Can you work these out from the model? Positions are in its coordinate system, mm. Face numbers are marked on the shaded views. A direction names the side the tool comes from. Coordinates: 2 decimals unless noted, no trailing zeros. Write each loop counter-clockwise with the first axis right and the second up, starting at its lowest first coordinate (ties: lowest second). Pieces come first, ordered by that corner, then holes. Notation, with made-up numbers: (33, 71.5) - (68, 71.5) arc R24 ccw to (68, 103.5) - close; hole circle Ø11 at (55, 56.5). An arc over 180 degrees is marked (long way). One line per question, with ' | ' between items. Start each with the question number.
from build123d import *

# Parameters (mm, degrees)
SKETCH1_W                  = 231.4
SKETCH1_H                  = 30
BOSS_EXTRUDE1_DEPTH        = 3
BOSS_EXTRUDE2_DEPTH        = 3
F_8_0_8_DIAMETER_HOLE1_D   = 8
F_10_0_10_DIAMETER_HOLE1_D = 10
F_6_0_6_DIAMETER_HOLE1_D   = 6


with BuildPart() as part:
    # Sketch1 → Boss-Extrude1 (new body)
    with BuildSketch(Plane.XY):
        with Locations((0, -15)):
            Rectangle(SKETCH1_W, SKETCH1_H)
    extrude(amount=BOSS_EXTRUDE1_DEPTH)

    # Sketch2 → Boss-Extrude2 (add)
    with BuildSketch(Plane(origin=(0, 0, 0), x_dir=(1, 0, 0), z_dir=(0, 1, 0))):
        Polygon((-115.7, -3), (115.7, -3), (85.7, -33), (-85.7, -33), align=None)
    extrude(amount=-BOSS_EXTRUDE2_DEPTH)

    # Ø8.0 (8) Diameter Hole1 (through all)
    with Locations(Plane(origin=(0, 0, 0), x_dir=(-1, 0, 0), z_dir=(0, 0, -1))):
        with Locations((-100.7, -15), (100.7, -15)):
            Hole(F_8_0_8_DIAMETER_HOLE1_D / 2)

    # Ø10.0 (10) Diameter Hole1 (through all)
    with Locations(Plane(origin=(0, 0, 0), x_dir=(-1, 0, 0), z_dir=(0, 0, -1))):
        with Locations((62.5, -15)):
            Hole(F_10_0_10_DIAMETER_HOLE1_D / 2)

    # Ø6.0 (6) Diameter Hole1 (through all)
    with Locations(Plane(origin=(0, 0, 0), x_dir=(1, 0, 0), z_dir=(0, 1, 0))):
        with Locations((0, -18)):
            Hole(F_6_0_6_DIAMETER_HOLE1_D / 2)


solid = part.part
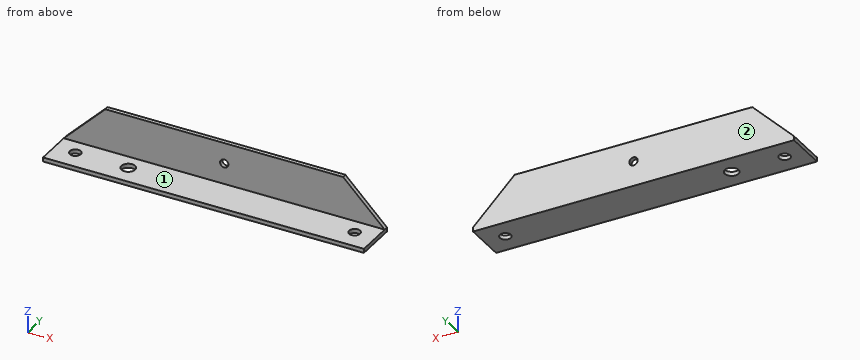
(1) I'm going to push flat-ended pins straight in: pin 1 (16 mm diameter, centred on x = -62.5, y = -15, fed in from +Z); pin 2 (12 mm diameter, centred on x = -55, z = 13.5, fed in from -Y). Where does each tip first touch, or does it pass through?
(2) If we section it at B-B on x = 0: List the corners of the cut face in (y, z) for me, plus the area to 3 significant figures.
(3) Which directions (+Z, -Z, +X, -X, +Y, -Y) give clear straight access to the entire face, cutting with the end or side of a thin tool? Please do the marked faces 1 and 2.
(4) If we section it at A-A on z = 18: List the corners of the cut face in (x, y) for me, plus the area to 3 significant figures.
(5) If I drill on probe 1 along Z at (x, y) = (0, -2.25); probe 2 along Z at (x, y) = (20.5, -22.5); probe 3 along Y at (x, z) = (27, 16), over which ranges is the centre line in solid material (lowest first)?
(6) If we section it at D-D on x = -100.7: List the corners of the cut face in (y, z) for me, plus the area to 3 significant figures.
(7) If we section it at C-C on y = -15: List the corners of the cut face in (x, z) for me, plus the area to 3 significant figures.
Values:
1) pin 1: z = 3 | pin 2: y = -3
2) outline: (-30, 0) - (0, 0) - (0, 15) - (-3, 15) - (-3, 3) - (-30, 3) - close; (-3, 21) - (0, 21) - (0, 33) - (-3, 33) - close | area: 162 mm2
3) face 1: +Z, +X, -X, -Y | face 2: +Z, -Z, +X, -X, +Y
4) outline: (-100.7, -3) - (-3, -3) - (-3, 0) - (-100.7, 0) - close; (3, -3) - (100.7, -3) - (100.7, 0) - (3, 0) - close | area: 586 mm2
5) probe 1: 0 to 15, 21 to 33 | probe 2: 0 to 3 | probe 3: -3 to 0
6) outline: (-30, 0) - (-19, 0) - (-19, 3) - (-30, 3) - close; (-11, 0) - (0, 0) - (0, 18) - (-3, 18) - (-3, 3) - (-11, 3) - close | area: 111 mm2
7) outline: (-115.7, 0) - (-104.7, 0) - (-104.7, 3) - (-115.7, 3) - close; (-96.7, 0) - (-67.5, 0) - (-67.5, 3) - (-96.7, 3) - close; (-57.5, 0) - (96.7, 0) - (96.7, 3) - (-57.5, 3) - close; (104.7, 0) - (115.7, 0) - (115.7, 3) - (104.7, 3) - close | area: 616 mm2
